Here's how the part is built. I have some questions about the finished solid (model axes, mm). Face numbers are marked on the shaded views. Give positions to 0.01 mm unless a question says otherwise; leave off trailing zeros. Loops run counter-clockwise (first coordinate to the right, second up) from the corner with the lowest first, then second, coordinate; pieces in that order, holes last. Notation, with made-up numbers: (25, 63.25) -> (60, 63.25) arc R19 cw to (60, 82.25) -> close; hole circle Ø3 at (76.5, 9). An arc over 180 degrees is marked (long way). Answer in a Markdown table with one row per item. Add a question column.
Item 1: We'd pull the mould along Y, two halves only. Please class the marked faces 1 and 2: released by +Y, released by -Y, zero draft, split by the parting line, or undercut.
Item 2: For P1, Ø10, axis at x = 2.5, y = 31.5, coming from the -Z side; P2, Ø3, axis at y = -7, z = 6, coming from the +X side; P3, Ø3, axis at x = -35, z = 6, coming from the +Y side; P4, Ø1, axis at x = -21, y = -5, coming from the +Z side, each with a flat end and sliding along its axis, tell me the tip position at first contact or that it passes through.
Item 3: If we section it at B-B (x = -35): Write out the boundary of the cut face in (y, z), then the cut area to 3 significant figures.
Item 4: If we section it at A-A (y = 0): Write out the boundary of the cut face in (x, z).
Item 5: If I drill on line 1 (X direction, y = 42.2, z = 6); line 2 (Y direction, x = -37, z = 6.5); line 3 (Z direction, x = -42.05, y = 0), over which ranges is the centre line in solid material (lowest first)?
Item 6: If we section it at D-D (x = 0): Write out the boundary of the cut face in (y, z).
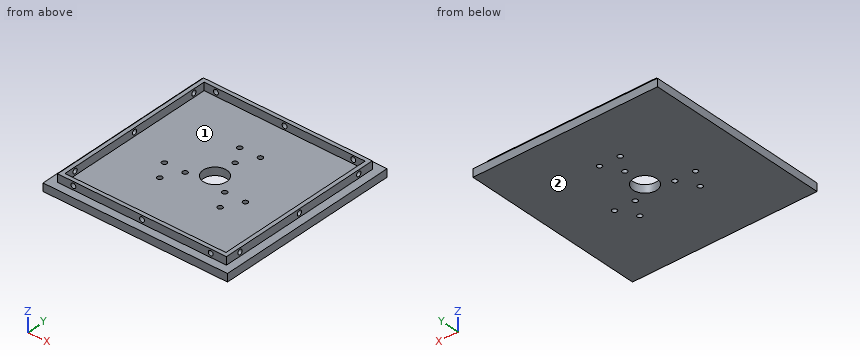
```python
from build123d import *

# Parameters (mm, degrees)
SKETCH_1_R               = 1.25
SKETCH_1_R_2             = 6
EXTRUDE_1_DEPTH          = 4
SKETCH_3_W               = 2
SKETCH_3_H               = 4
EXTRUDE_2_DEPTH          = 43
SKETCH_4_W               = 4
SKETCH_4_H               = 2
EXTRUDE_3_DEPTH          = 43
SKETCH_5_R               = 1.25
CUT_EXTRUDE_1_DEPTH      = 2
PATTERN_CIRCULAR_1_COUNT = 4


with BuildPart() as part:
    # 草图1 → 凸台-拉伸1 (new body)
    with BuildSketch(Plane.XY):
        Polygon((47, 47), (0, 47), (-47, 47), (-47, 0), (-47, -47), (0, -47), (47, -47), (47, 0), align=None)
        with Locations((-15.266370453, -14.873586171)):
            Circle(SKETCH_1_R, mode=Mode.SUBTRACT)
        with Locations((-20.618803135, -5.965642279)):
            Circle(SKETCH_1_R, mode=Mode.SUBTRACT)
        with Locations((-10.228081088, -5.784271551)):
            Circle(SKETCH_1_R, mode=Mode.SUBTRACT)
        with Locations((15.47579933, -14.873586171)):
            Circle(SKETCH_1_R, mode=Mode.SUBTRACT)
        with Locations((10.123366649, -5.965642279)):
            Circle(SKETCH_1_R, mode=Mode.SUBTRACT)
        with Locations((20.514088696, -5.784271551)):
            Circle(SKETCH_1_R, mode=Mode.SUBTRACT)
        with Locations((-5.247718243, 20.657857721)):
            Circle(SKETCH_1_R, mode=Mode.SUBTRACT)
        Circle(SKETCH_1_R_2, mode=Mode.SUBTRACT)
        with Locations((0.104714439, 11.749913829)):
            Circle(SKETCH_1_R, mode=Mode.SUBTRACT)
        with Locations((5.143003804, 20.839228449)):
            Circle(SKETCH_1_R, mode=Mode.SUBTRACT)
    extrude(amount=EXTRUDE_1_DEPTH)

    # 草图3 → 凸台-拉伸2 (add, symmetric)
    with BuildSketch(Plane(origin=(0, 0, 0), x_dir=(1, 0, 0), z_dir=(0, 1, 0))):
        with Locations((-42, -6)):
            Rectangle(SKETCH_3_W, SKETCH_3_H)
        with Locations((42, -6)):
            Rectangle(SKETCH_3_W, SKETCH_3_H)
    extrude(amount=EXTRUDE_2_DEPTH, both=True)

    # 草图4 → 凸台-拉伸3 (add, symmetric)
    with BuildSketch(Plane(origin=(0, 0, 0), x_dir=(0, 0, -1), z_dir=(1, 0, 0))):
        with Locations((-6, -42)):
            Rectangle(SKETCH_4_W, SKETCH_4_H)
        with Locations((-6, 42)):
            Rectangle(SKETCH_4_W, SKETCH_4_H)
    extrude(amount=EXTRUDE_3_DEPTH, both=True)

    # 草图5 → 切除-拉伸1 (cut)
    with BuildSketch(Plane(origin=(0, 43, 0), x_dir=(1, 0, 0), z_dir=(0, 1, 0))):
        with Locations((0, -6)):
            Circle(SKETCH_5_R)
        with Locations((35, -6)):
            Circle(SKETCH_5_R)
        with Locations((-35, -6)):
            Circle(SKETCH_5_R)
    cut_extrude_1 = extrude(amount=-CUT_EXTRUDE_1_DEPTH, mode=Mode.SUBTRACT)

    # 阵列(圆周)1: 切除-拉伸1 ×4 about axis
    pattern_circular_1_axis = Axis((0, 0, 4), (0, 0, 1))
    for i in range(1, PATTERN_CIRCULAR_1_COUNT):
        add(cut_extrude_1.rotate(pattern_circular_1_axis, i * 360 / PATTERN_CIRCULAR_1_COUNT), mode=Mode.SUBTRACT)


solid = part.part
```
Recorded:
| question | item | result |
|---|---|---|
| 1 | face 1 | undercut |
| 1 | face 2 | zero draft |
| 2 | P1 | stops at z = 0 |
| 2 | P2 | stops at x = 43 |
| 2 | P3 | stops at y = 43 |
| 2 | P4 | stops at z = 4 |
| 3 | outline | (-47, 0) -> (47, 0) -> (47, 4) -> (43, 4) -> (43, 4.75) -> (41, 4.75) -> (41, 4) -> (-41, 4) -> (-41, 4.75) -> (-43, 4.75) -> (-43, 4) -> (-47, 4) -> close; (-43, 7.25) -> (-41, 7.25) -> (-41, 8) -> (-43, 8) -> close; (41, 7.25) -> (43, 7.25) -> (43, 8) -> (41, 8) -> close |
| 3 | area | 382 mm^2 |
| 4 | outline | (-47, 0) -> (-6, 0) -> (-6, 4) -> (-41, 4) -> (-41, 4.75) -> (-43, 4.75) -> (-43, 4) -> (-47, 4) -> close; (-43, 7.25) -> (-41, 7.25) -> (-41, 8) -> (-43, 8) -> close; (6, 0) -> (47, 0) -> (47, 4) -> (43, 4) -> (43, 4.75) -> (41, 4.75) -> (41, 4) -> (6, 4) -> close; (41, 7.25) -> (43, 7.25) -> (43, 8) -> (41, 8) -> close |
| 5 | line 1 | x = -43 to -36.25, -33.75 to -1.25, 1.25 to 33.75, 36.25 to 43 |
| 5 | line 2 | y = -43 to -41, 41 to 43 |
| 5 | line 3 | z = 0 to 4.75, 7.25 to 8 |
| 6 | outline | (-47, 0) -> (-6, 0) -> (-6, 4) -> (-41, 4) -> (-41, 4.75) -> (-43, 4.75) -> (-43, 4) -> (-47, 4) -> close; (-43, 7.25) -> (-41, 7.25) -> (-41, 8) -> (-43, 8) -> close; (6, 0) -> (10.5, 0) -> (10.5, 4) -> (6, 4) -> close; (13, 0) -> (47, 0) -> (47, 4) -> (43, 4) -> (43, 4.75) -> (41, 4.75) -> (41, 4) -> (13, 4) -> close; (41, 7.25) -> (43, 7.25) -> (43, 8) -> (41, 8) -> close |
